```python
from build123d import *

# Parameters (mm, degrees)
SKETCH1_R           = 45
BOSS_EXTRUDE1_DEPTH = 3
SKETCH2_W           = 35
SKETCH2_H           = 24
CUT_EXTRUDE1_DEPTH  = 3
CHAMFER1_SIZE       = 2
SKETCH3_W           = 36
SKETCH3_H           = 34
CUT_EXTRUDE2_DEPTH  = 2


with BuildPart() as part:
    # Sketch1 → Boss-Extrude1 (new body)
    with BuildSketch(Plane.XY):
        Circle(SKETCH1_R)
    extrude(amount=BOSS_EXTRUDE1_DEPTH)

    # Sketch2 → Cut-Extrude1 (cut)
    with BuildSketch(Plane.XY.offset(3)):
        Rectangle(SKETCH2_W, SKETCH2_H)
    extrude(amount=-CUT_EXTRUDE1_DEPTH, mode=Mode.SUBTRACT)

    # Chamfer1
    chamfer1_edges = [part.edges().sort_by_distance(p)[0] for p in [
        (-45, 0, 3),
    ]]
    chamfer(chamfer1_edges, length=CHAMFER1_SIZE)

    # Sketch3 → Cut-Extrude2 (cut)
    with BuildSketch(Plane(origin=(0, 0, 0), x_dir=(-1, 0, 0), z_dir=(0, 0, -1))):
        Rectangle(SKETCH3_W, SKETCH3_H)
    extrude(amount=-CUT_EXTRUDE2_DEPTH, mode=Mode.SUBTRACT)


solid = part.part
```
Input: part model. Units: mm. Frame: model coordinates. A direction names the side the tool comes from. Coordinates: 2 decimals unless noted, no trailing zeros. Loops run counter-clockwise (first coordinate to the right, second up) from the corner with the lowest first, then second, coordinate; pieces in that order, holes last.
Q1. Section B-B, the plane y = 0. Return the cut outline in (x, z).
Results are:
outline: (-45, 0) - (-18, 0) - (-18, 2) - (-17.5, 2) - (-17.5, 3) - (-43, 3) - (-45, 1) - close; (17.5, 2) - (18, 2) - (18, 0) - (45, 0) - (45, 1) - (43, 3) - (17.5, 3) - close
Q2. Mould query, pull axis Y, two halves, no side actions, for faces 3 (the flat face through (-18, 0, 1)), 4 (the flat face through (1, -13, 2)), 5 (the flat face through (19, 1, 3)), 6 (the cylindrical face through (20.765, -39.923, 0.493)). Classes: +Y half, -Y half, draft (parallel to the pull), parting line (faces both ways), or undercut.
Results are:
face 3: undercut
face 4: undercut
face 5: draft
face 6: parting line
Q3. Contact query for flat-ended pins moving along their axis: pin 1 (0.8 mm diameter, centred on y = 2.5, z = 2.5, fed in from +X); pin 2 (1.6 mm diameter, centred on y = -2, z = 1.5, fed in from -X); pin 3 (1.1 mm diameter, centred on x = -3.5, z = 2.5, fed in from -Y). Output: stop coordinate, or through.
Results are:
pin 1: stops at x = 43.83
pin 2: stops at x = -44.98
pin 3: stops at y = -43.91
Q4. Section A-A, the plane x = 0. Return the cut outline in (y, z).
Results are:
outline: (-45, 0) - (-17, 0) - (-17, 2) - (-12, 2) - (-12, 3) - (-43, 3) - (-45, 1) - close; (12, 2) - (17, 2) - (17, 0) - (45, 0) - (45, 1) - (43, 3) - (12, 3) - close
Q5. Line query: line 1 along X through (y, z) = (-11.5, 0.85); line 2 along X through (y, z) = (-12.5, 0.95); line 3 along Y through (x, z) = (-8, 0.7). Output: solid intervals per line, ascending.
Results are:
line 1: x = -43.51 to -18, 18 to 43.51
line 2: x = -43.23 to -18, 18 to 43.23
line 3: y = -44.28 to -17, 17 to 44.28
Q6. Set-up query: faces 1 (the flat face through (19, 1, 0)), 2 (the flat face through (0, 17, 1)). Return all of +Z, -Z, +X, -X, +Y, -Y with unobstructed straight access to the full face (end or side cutting, diameter ignored); none if empty.
Results are:
face 1: -Z, +X, -X, +Y, -Y
face 2: -Z
